Answer from the drawing. Dimensions are ordinates in mm from the lowest x, y and z of the part. Round coordinates to 2 decimals unless told otherwise and drop trailing zeros. Loops run counter-clockwise (first coordinate to the right, second up) from the corner with the lowest first, then second, coordinate; pieces in that order, holes last. Notation, with made-up numbers: M 89,39 L 94,39 A13 ccw 94,56 Z; hole C 37,57.5 d6. An arc over 180 degrees is marked long. Answer as a JSON object with one key per item and string values.
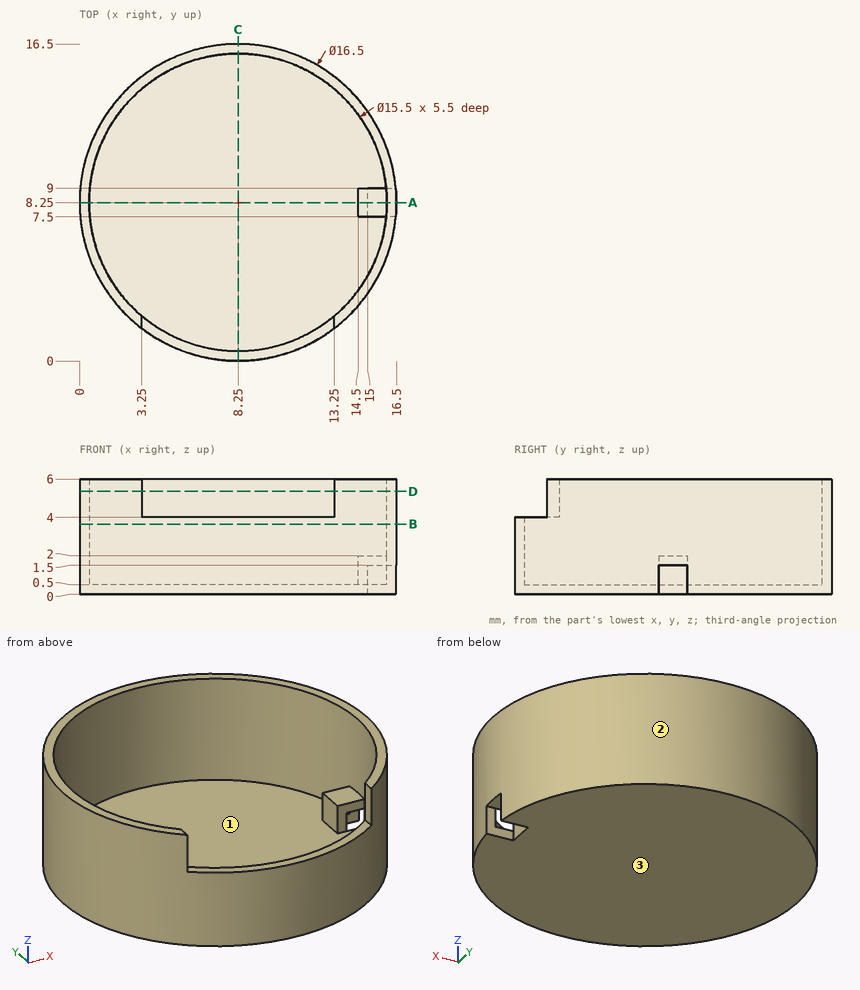
Item 1: Straight lines are drawn through the part: line 1 (X direction, y = 8.25, z = 2.9); line 2 (X direction, y = 8.25, z = 1.65). For each, find the intervals that lie inside material, in ascending order.
Values follow:
{"line 1": "0 to 0.5, 16 to 16.5", "line 2": "0 to 0.5, 14.5 to 16.5"}
Item 2: Flat-ended cylindrical pins translate along their axes: P1, Ø0.8, axis at x = 16, y = 8, coming from the -Z side; P2, Ø0.7, axis at x = 10, y = 1, coming from the +Z side; P3, Ø1, axis at x = 8, y = 12, coming from the +Z side. Find the tip coordinate at first contact, or state that the pin passes through.
Values follow:
{"P1": "z = 1.5", "P2": "z = 4", "P3": "z = 0.5"}
Item 3: The part is cut by section D-D (z = 5.35). Give the vertices of the cut face in (x, y).
Values follow:
{"outline": "M 3.25,1.69 L 3.25,2.33 A7.75 cw long 13.25,2.33 L 13.25,1.69 A8.25 ccw long Z"}
Item 4: The part is cut by section C-C (x = 8.25). Give the vertices of the cut face in (y, z).
Values follow:
{"outline": "M 0,0 L 16.5,0 L 16.5,6 L 16,6 L 16,0.5 L 0.5,0.5 L 0.5,4 L 0,4 Z"}
Item 5: The part is cut by section B-B (z = 3.65). Give the vertices of the cut face in (x, y).
Values follow:
{"outline": "C 8.25,8.25 d16.5; hole C 8.25,8.25 d15.5"}
Item 6: The part is cut by section A-A (y = 8.25). Give the vertices of the cut face in (x, z), then the cut area to 4 significant figures.
Values follow:
{"outline": "M 0,0 L 15,0 L 15,1.5 L 16.5,1.5 L 16.5,6 L 16,6 L 16,2 L 14.5,2 L 14.5,0.5 L 0.5,0.5 L 0.5,6 L 0,6 Z", "area": "13.75 mm^2"}
Item 7: Determine the mould class of the marked faces 1, 2 and 3 for opening direction X: released by +X, released by -X, zero draft, split by the parting line, or undercut.
Values follow:
{"face 1": "undercut", "face 2": "split by the parting line", "face 3": "zero draft"}
